from build123d import *

# Parameters (mm, degrees)
F3_DEPTH = 2.8
F4_W     = 15.5
F4_H     = 60
F5_DEPTH = 25
F7_DEPTH = 0.4
F8_R     = 6
F9_R     = 0.5
F10_R    = 3


# Not quite as in the source:
# - a pattern or mirror of a feature is missing from the dataset's text; its kind, count and spacing are read off the source's solid


with BuildPart() as f3:
    # F2 (on Top) → F3 (new body)
    with BuildSketch(Plane.XY):
        with BuildLine():
            Line((4.5, -32.5), (17.75, -32.5))
            Line((17.75, -32.5), (17.75, 32.5))
            Line((17.75, 32.5), (-17.75, 32.5))
            Line((-17.75, 32.5), (-17.75, -32.5))
            Line((-17.75, -32.5), (-4.5, -32.5))
            Line((-4.5, -32.5), (-4.5, 2.5))
            ThreePointArc((-4.5, 2.5), (0, 7), (4.5, 2.5))
            Line((4.5, 2.5), (4.5, -32.5))
        make_face()
    extrude(amount=F3_DEPTH)

    # F4 (on offset) → F5 (cut)
    with BuildSketch(Plane.XY.offset(1.8)):
        with Locations((0, -2.5)):
            Rectangle(F4_W, F4_H)
    extrude(amount=F5_DEPTH, mode=Mode.SUBTRACT)

    # F6 (on face) → F7 (cut)
    with BuildSketch(Plane.XY.offset(2.8)):
        with BuildLine():
            Line((9.25, 2), (16.25, 2))
            ThreePointArc((16.25, 2), (16.75, 2.5), (16.25, 3))
            Line((16.25, 3), (9.25, 3))
            ThreePointArc((9.25, 3), (8.75, 2.5), (9.25, 2))
        make_face()
    f7 = extrude(amount=-F7_DEPTH, mode=Mode.SUBTRACT)

    # F7_copies: F7 across plane
    add(f7.mirror(Plane(origin=(0, 0, 0), x_dir=(0, 0, -1), z_dir=(-1, 0, 0))), mode=Mode.SUBTRACT)

    # F8
    f8_edges = [f3.edges().sort_by_distance(p)[0] for p in [
        (-17.75, -32.5, 1.4),
        (17.75, -32.5, 1.4),
        (-17.75, 32.5, 1.4),
        (17.75, 32.5, 1.4),
    ]]
    fillet(f8_edges, radius=F8_R)

    # F9
    f9_edges = [f3.edges().sort_by_distance(p)[0] for p in [
        (7.75, 27.5, 2.3),
        (-7.75, 27.5, 2.3),
    ]]
    fillet(f9_edges, radius=F9_R)

    # F10
    f10_edges = [f3.edges().sort_by_distance(p)[0] for p in [
        (7.75, -32.5, 2.3),
        (-7.75, -32.5, 2.3),
        (-4.5, -32.5, 0.9),
        (4.5, -32.5, 0.9),
    ]]
    fillet(f10_edges, radius=F10_R)


solid = f3.part
Check sheet for the modelled part. Datum: model origin and axes. Units: mm. A direction names the side the tool comes from. Round coordinates to 2 decimals unless told otherwise and drop trailing zeros. Write each loop counter-clockwise with the first axis right and the second up, starting at its lowest first coordinate (ties: lowest second). Pieces come first, ordered by that corner, then holes. Notation, with made-up numbers: (34.5, -38.5) -> (85.5, -38.5) arc R9 ccw to (85.5, -26.5) -> close; hole circle Ø5 at (62.25, 0.25). An arc over 180 degrees is marked (long way). Answer as CSV lines item,"result". Start each with the question number.
1) Section check A-A on y = -18. Enter the section's corners in (x, z), and give its area (3 significant figures).
2) Section check C-C on z = 1.1. Enter the section's corners in (x, y), and give its area (3 significant figures).
3) Material ranges on line 1 (X direction, y = -4, z = 1); line 2 (X direction, y = 15, z = 1.9); line 3 (Y direction, x = 4.5, z = 1.85), recorded low to high. Write a range as from..to.
4) Go/stop test with flat-tipped pins: P1, Ø0.8, axis at x = 13, y = 2.5, coming from the +Z side; P2, Ø1.1, axis at x = 3, z = 2.5, coming from the -Y side; P3, Ø6.5, axis at x = -2, y = -15, coming from the +Z side. Record where each tip stops, or that it passes through.
5) Section check B-B on y = 15. Enter the section's corners in (x, z), and give its area (3 significant figures).
6) Tool access check on faces 1 (the cylindrical face through (5.4, -31.64, 0.91)), 2 (the cylindrical face through (8.61, -31.6, 2.31)), 3 (the cylindrical face through (-16.039, -30.696, 1.42)). Record the directions out of +Z, -Z, +X, -X, +Y, -Y that give a thin tool (end or side, any length) a straight path to the whole face; none if there is none.
7) Section check D-D on x = 0. Enter the section's corners in (y, z), and give its area (3 significant figures).
8) Release check for a two-part mould opening along X. For faces 4 (the flat face through (4.5, -13, 1)), 5 (the flat face through (0, 32.5, 1)), 6 (the flat face through (-17.75, 0, 1)) record: pulls with the +X half, pulls with the -X half, needs draft (parallel to the pull), parting line crosses it, or undercut.
Found:
1,outline,"(-17.75, 0) -> (-4.5, 0) -> (-4.5, 1.8) -> (-7.75, 1.8) -> (-7.75, 2.8) -> (-17.75, 2.8) -> close; (4.5, 0) -> (17.75, 0) -> (17.75, 2.8) -> (7.75, 2.8) -> (7.75, 1.8) -> (4.5, 1.8) -> close"
1,area,"67.7 mm^2"
2,outline,"(-17.75, -26.5) arc R6 ccw to (-11.75, -32.5) -> (-7.5, -32.5) arc R3 ccw to (-4.5, -29.5) -> (-4.5, 2.5) arc R4.5 cw to (4.5, 2.5) -> (4.5, -29.5) arc R3 ccw to (7.5, -32.5) -> (11.75, -32.5) arc R6 ccw to (17.75, -26.5) -> (17.75, 26.5) arc R6 ccw to (11.75, 32.5) -> (-11.75, 32.5) arc R6 ccw to (-17.75, 26.5) -> close"
2,area,"1,930 mm^2"
3,line 1,"x = -17.75..-4.5, 4.5..17.75"
3,line 2,"x = -17.75..-7.75, 7.75..17.75"
3,line 3,"y = 27.5..32.5"
4,P1,"stops at z = 2.4"
4,P2,"stops at y = 27.5"
4,P3,"stops at z = 1.8"
5,outline,"(-17.75, 0) -> (17.75, 0) -> (17.75, 2.8) -> (7.75, 2.8) -> (7.75, 1.8) -> (-7.75, 1.8) -> (-7.75, 2.8) -> (-17.75, 2.8) -> close"
5,area,"83.9 mm^2"
6,face 1,"+Z, -Z, -Y"
6,face 2,"+Z, -Y"
6,face 3,"+Z, -Z, -X, -Y"
7,outline,"(7, 0) -> (32.5, 0) -> (32.5, 2.8) -> (27.5, 2.8) -> (27.5, 1.8) -> (7, 1.8) -> close"
7,area,"50.9 mm^2"
8,face 4,"undercut"
8,face 5,"needs draft"
8,face 6,"pulls with the -X half"
